Part print with two shaded views. Sizes in mm from the minimum x, y, z corner. A direction names the side the tool comes from. Give positions to 0.01 mm unless a question says otherwise; leave off trailing zeros. Write each loop counter-clockwise with the first axis right and the second up, starting at its lowest first coordinate (ties: lowest second). Pieces come first, ordered by that corner, then holes.
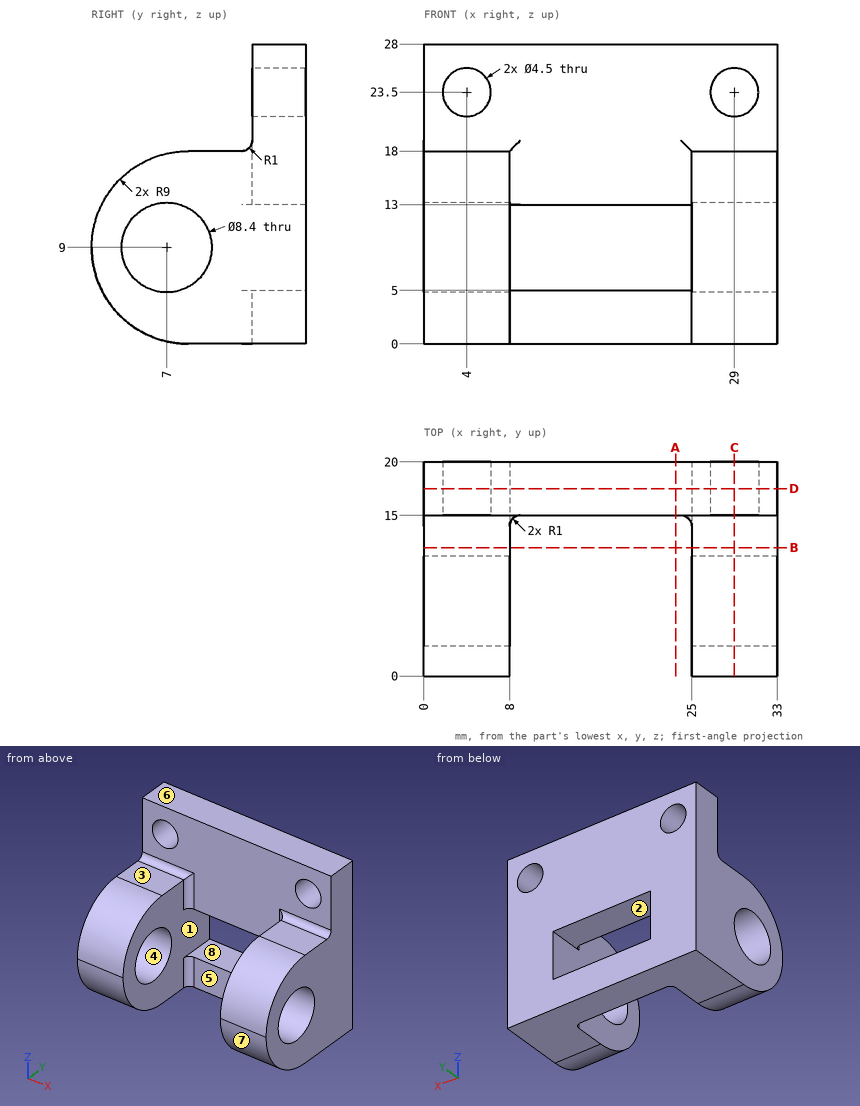
1) Saw through at C-C, the plane x = 29. Count the separate pieces of the cut face and the enclosed holes in it, then the cut area to 3 significant figures.
Answers follow:
separate pieces: 2
enclosed holes: 1
area: 298 mm2
2) Pin check, flat tips, straight feed: pin 1 Ø4 at (x, z) = (14.5, 18) entering from -Y; pin 2 Ø5 at (y, z) = (7, 9) entering from -X; pin 3 Ø1.5 at (x, y) = (4, 11.5) entering from +Z. Stop position of each tip, or through.
Answers follow:
pin 1: stops at y = 15
pin 2: passes through
pin 3: stops at z = 18
3) Wall check: L1, parallel to X at y = 17.6, z = 23.5; L2, parallel to X at y = 9.5, z = 5; L3, parallel to Z at x = 14, y = 16.5. Give the ranges that are in metal, low to high.
Answers follow:
L1: x = 0 to 1.75, 6.25 to 26.75, 31.25 to 33
L2: x = 0 to 8, 25 to 33
L3: z = 0 to 5, 13 to 28
4) Two-plate mould, pull along Z, no slides. Class the marked faces 6, 7 and 8: +Z half, -Z half, draft (parallel to the pull), parting line (faces both ways), or undercut.
Answers follow:
face 6: +Z half
face 7: -Z half
face 8: undercut
5) Saw through at A-A, the plane x = 23.5. Write the cut outline in (y, z).
Answers follow:
outline: (15, 0) - (20, 0) - (20, 5) - (15, 5) - close; (15, 13) - (20, 13) - (20, 28) - (15, 28) - close
6) Saw through at D-D, the plane y = 17.5. Write the cut outline in (x, z).
Answers follow:
outline: (0, 0) - (33, 0) - (33, 28) - (0, 28) - close; hole circle Ø4.5 at (4, 23.5); hole (8, 5) - (25, 5) - (25, 13) - (8, 13) - close; hole circle Ø4.5 at (29, 23.5)
7) Saw through at B-B, the plane y = 12. Write the cut outline in (x, z).
Answers follow:
outline: (0, 0) - (8, 0) - (8, 18) - (0, 18) - close; (25, 0) - (33, 0) - (33, 18) - (25, 18) - close
8) 3-axis set-ups, long thin cutter, end or side, ignore diameter. For the marked faces 1, 2, 3, 4 and 5: which of +Z, -Z, +X, -X, +Y, -Y reach the whole face in a straight line?
Answers follow:
face 1: -Y
face 2: +Y, -Y
face 3: +Z, +X, -X, -Y
face 4: +X, -X
face 5: +Z, -Z, -Y
